Job drawing, mm, ordinate dimensions from the low corner. One solid piece. Round coordinates to 2 decimals unless told otherwise and drop trailing zeros. Order: outer loops, then holes, each group sorted by start corner. A loop starts at its lowest first (then second) coordinate and runs counter-clockwise, first axis right, second up. Notation, with made-up numbers: (15, 30.25) - (49, 30.25) arc R30 cw to (49, 64.25) - close; hole circle Ø1 at (47.25, 70). An arc over 180 degrees is marked (long way). Use one line per item in the form item = value. Start each with the question number.
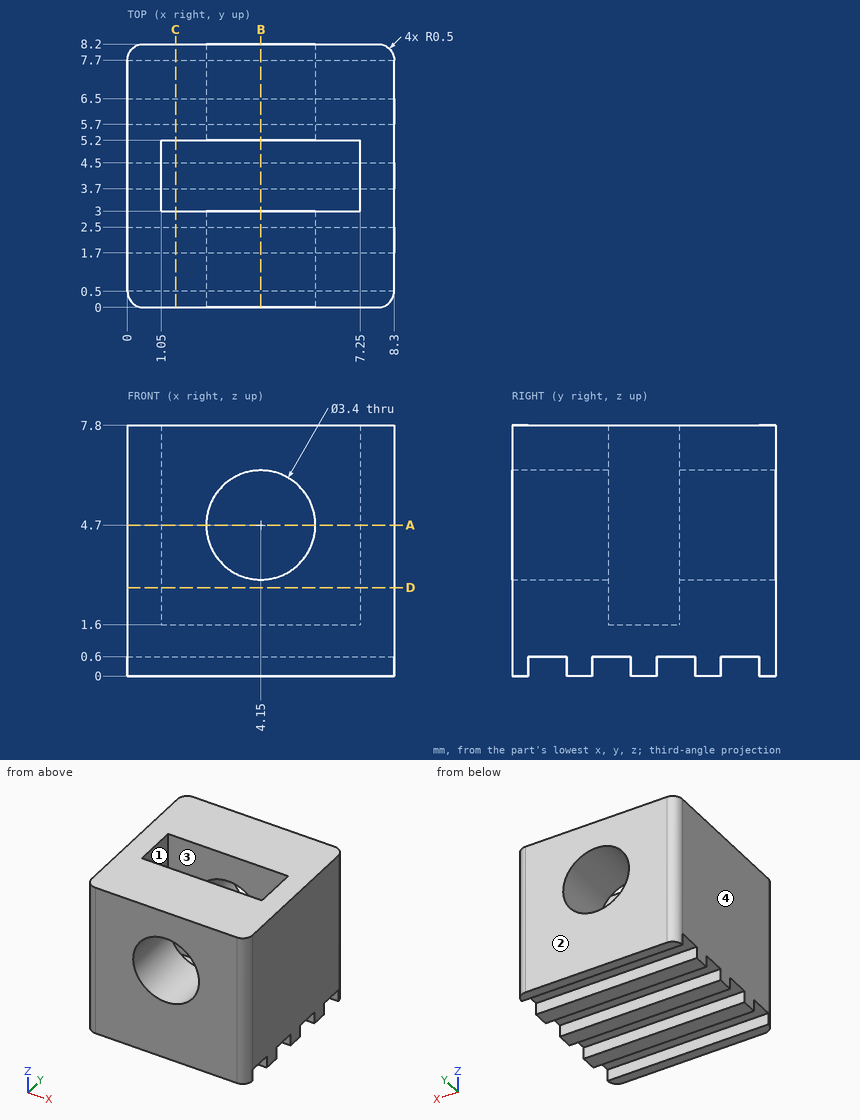
(1) Slice it at B-B (x = 4.15). Give the number of separate pieces and of enclosed holes in the cut face, and give its area (3 significant figures).
(2) Mould opens along Y. For the marked faces 1, 2, 3 and 4 say: pulls with the +Y half, pulls with the -Y half, needs draft (parallel to the pull), parting line crosses it, or undercut.
(3) Slice it at A-A (z = 4.7). Give the cut face in (x, y).
(4) Slice it at D-D (z = 2.75). Give the cut face in (x, y), and give its area (3 significant figures).
(5) Slice it at C-C (x = 1.5). Give the cut face in (y, z).
(6) Flat gauge pins, fed straight in: P1, Ø1, axis at y = 5, z = 1.5, coming from the -X side; P2, Ø3, axis at x = 4.15, z = 4.7, coming from the +Y side. Where does each tip first touch, or does it go through?
(7) Wall check: line 1 (Y direction, x = 2.25, z = 1.75); line 2 (X direction, y = 4.25, z = 7.25); line 3 (X direction, y = 1.15, z = 4.7). Give the ranges that are in metal, low to high. Write a range as [from, to].
Results list:
q1.separate_pieces = 3
q1.enclosed_holes = 0
q1.area = 27.0 mm²
q2.face_1 = undercut
q2.face_2 = pulls with the +Y half
q2.face_3 = undercut
q2.face_4 = needs draft
q3.outline = (0, 0.5) arc R0.5 ccw to (0.5, 0) - (2.45, 0) - (2.45, 3) - (1.05, 3) - (1.05, 5.2) - (2.45, 5.2) - (2.45, 8.2) - (0.5, 8.2) arc R0.5 ccw to (0, 7.7) - close; (5.85, 0) - (7.8, 0) arc R0.5 ccw to (8.3, 0.5) - (8.3, 7.7) arc R0.5 ccw to (7.8, 8.2) - (5.85, 8.2) - (5.85, 5.2) - (7.25, 5.2) - (7.25, 3) - (5.85, 3) - close
q4.outline = (0, 0.5) arc R0.5 ccw to (0.5, 0) - (7.8, 0) arc R0.5 ccw to (8.3, 0.5) - (8.3, 7.7) arc R0.5 ccw to (7.8, 8.2) - (0.5, 8.2) arc R0.5 ccw to (0, 7.7) - close; hole (1.05, 3) - (7.25, 3) - (7.25, 5.2) - (1.05, 5.2) - close
q4.area = 54.2 mm²
q5.outline = (0, 0) - (0.5, 0) - (0.5, 0.6) - (1.7, 0.6) - (1.7, 0) - (2.5, 0) - (2.5, 0.6) - (3.7, 0.6) - (3.7, 0) - (4.5, 0) - (4.5, 0.6) - (5.7, 0.6) - (5.7, 0) - (6.5, 0) - (6.5, 0.6) - (7.7, 0.6) - (7.7, 0) - (8.2, 0) - (8.2, 7.8) - (5.2, 7.8) - (5.2, 1.6) - (3, 1.6) - (3, 7.8) - (0, 7.8) - close
q6.P1 = 0
q6.P2 = through
q7.line_1 = [0, 3], [5.2, 8.2]
q7.line_2 = [0, 1.05], [7.25, 8.3]
q7.line_3 = [0, 2.45], [5.85, 8.3]
